Model file for the job. Use its own axes, mm. A direction names the side the tool comes from. Give positions to 0.01 mm unless a question says otherwise; leave off trailing zeros. Loops run counter-clockwise (first coordinate to the right, second up) from the corner with the lowest first, then second, coordinate; pieces in that order, holes last. Notation, with made-up numbers: (-28.75, -32.5) - (16.25, -32.5) arc R38 cw to (16.25, 5.5) - close; hole circle Ø9 at (86, 78). An arc over 180 degrees is marked (long way). Use a Markdown table: item, result.
Autodesk Inventor part; units mm, degrees
ref_plane "YZ Plane" through (0, 0, 0) normal (1, 0, 0) x (0, 1, 0)
ref_plane "XZ Plane" through (0, 0, 0) normal (0, 1, 0) x (-1, 0, 0)
ref_plane "XY Plane" through (0, 0, 0) normal (0, 0, 1) x (1, 0, 0)
sketch "Sketch1" plane through (0, 0, 0) normal (0, 1, 0) x (-1, 0, 0)
  line L0 (17, 5) -> (-17, 5)
  line L1 (-17, 5) -> (-17, -5)
  line L2 (-17, -5) -> (17, -5)
  line L3 (17, -5) -> (17, 5)
  line L4 (17, 5) -> (-17, -5) construction
  line L5 (-17, 5) -> (17, -5) construction
  point P0 (0, 0)
  dimension "d0" = 34
  dimension "d1" = 10
extrude "Extrusion1" add sketch "Sketch1" along normal blind 2.5
sketch "Sketch2" plane through (0, 2.5, 0) normal (0, 1, 0) x (1, 0, 0)
  line L0 (-17, 5) -> (-17, -5)
  circle A0 centre (-17, 0) radius 5
  line L1 (17, -5) -> (17, 5)
  circle A1 centre (17, 0) radius 5
  point P0 (0, 0)
extrude "Extrusion2" add sketch "Sketch2" against normal blind 2.5
sketch "Sketch3" plane through (0, 2.5, 0) normal (0, 1, 0) x (1, 0, 0)
  arc A0 (-17, 5) -> (-17, -5) centre (-17, 0) ccw
  circle A1 centre (-17, 0) radius 1.5
  arc A2 (17, -5) -> (17, 5) centre (17, 0) ccw
  circle A3 centre (17, 0) radius 1.5
  point P0 (0, 0)
  dimension "d6" = 3
  dimension "d7" = 3
hole "Hole1" at (-17, 2.5, 0) at (17, 2.5, 0) direction (0, -1, 0) diameter 2.85 end through all
sketch "Sketch4" plane through (0, 2.5, 0) normal (0, 1, 0) x (1, 0, 0)
  circle A0 centre (-17, 0) radius 4.25
  arc A1 (-17, 5) -> (-17, -5) centre (-17, 0) ccw
  arc A2 (17, -5) -> (17, 5) centre (17, 0) ccw
  circle A3 centre (17, 0) radius 4.25
  point P0 (0, 0)
  dimension "d15" = 8.5
  dimension "d16" = 8.5
extrude "Extrusion3" cut sketch "Sketch4" against normal blind 0.5
sketch "Sketch5" plane through (0, 2.5, 0) normal (0, 1, 0) x (1, 0, 0)
  circle A0 centre (0, 5) radius 1.5
  circle A1 centre (0, -5) radius 1.5
  circle A2 centre (0, 13.5) radius 10
  point P0 (0, 0)
  dimension "d19" = 3
  dimension "d20" = 5
  dimension "d21" = 3
  dimension "d22" = 5
  dimension "d23" = 20
extrude "Extrusion4" cut sketch "Sketch5" against normal through all contours A0 | A2
mirror "Mirror1" about plane through (0, 0, 0) normal (0, 0, 1) of "Extrusion4"
sketch "Sketch6" plane through (0, 2.5, 0) normal (0, 1, 0) x (1, 0, 0)
  circle A0 centre (6, 0) radius 3
  point P0 (0, 0)
  dimension "d26" = 6
  dimension "d27" = 6
extrude "Extrusion5" cut sketch "Sketch6" against normal blind 0.5
sketch "Sketch7" plane through (6, 2, 0) normal (0, 1, 0) x (1, 0, 0)
  circle A0 centre (0, 0) radius 3
  circle A1 centre (0, 0) radius 1.5
  point P0 (-6, 0)
  dimension "d30" = 3
extrude "Extrusion6" cut sketch "Sketch7" against normal through all contours A1
mirror "Mirror2" about plane through (0, 0, 0) normal (1, 0, 0) of "Extrusion5", "Extrusion6"
fillet "Fillet1" radius 4 4 edges at (5.2678, 1.25, 5) (-5.2678, 1.25, 5) (5.2678, 1.25, -5) (-5.2678, 1.25, -5)
properties part number "Tarot-mr4008-blade-adapter"
(1) Mould opens along X. For faces 1 (the flat face through (0, 0, 0)), 2 (the cylindrical face through (22, 1, 0)), 3 (the flat face through (-4.7, 2, 1.3)) say: pulls with the +X half, pulls with the -X half, needs draft (parallel to the pull), parting line crosses it, or undercut.
Computed:
| item | result |
|---|---|
| face 1 | needs draft |
| face 2 | pulls with the +X half |
| face 3 | undercut |
(2) Drill centre lines: probe 1 along X at (y, z) = (0.6, 0) (3 decimals); probe 2 along Z at (x, y) = (-17, 1.35) (3 decimals); probe 3 along Z at (x, y) = (-17, 2.45). Where is each one in solid material? Low to high. Write a range as [from, to].
Computed:
| item | result |
|---|---|
| probe 1 | [-22, -18.425], [-15.575, -7.5], [-4.5, 4.5], [7.5, 15.575], [18.425, 22] |
| probe 2 | [-5, -1.425], [1.425, 5] |
| probe 3 | [-5, -4.25], [4.25, 5] |
(3) Pin check, flat tip, straight feed: P1, Ø2.5, axis at x = -18.5, z = -0.5, coming from the +Y side. Stop position of the tip, or through.
Computed:
| item | result |
|---|---|
| P1 | y = 2 |
(4) Slice it at D-D, the plane z = -0.75. Count the separate pieces of the cut face and the enclosed holes in it, plus the area to 3 significant figures.
Computed:
| item | result |
|---|---|
| separate pieces | 5 |
| enclosed holes | 0 |
| area | 75.5 mm² |
(5) 3-axis set-ups, long thin cutter, end or side, ignore diameter. For faces 4 (the flat face through (-17, 2, 2)), 5 (the cylindrical face through (5.392, 1.268, -4.894)), 6 (the cylindrical face through (-5.392, 1.268, 4.894)): which of +Z, -Z, +X, -X, +Y, -Y reach the whole face in a straight line?
Computed:
| item | result |
|---|---|
| face 4 | +Y |
| face 5 | -Z, +Y, -Y |
| face 6 | +Z, +Y, -Y |
(6) Slice it at B-B, the plane x = 15. Write the cut outline in (y, z), plus the area to 4 significant figures.
Computed:
| item | result |
|---|---|
| outline | (0, -5) - (2.5, -5) - (2.5, -3.75) - (2, -3.75) - (2, 3.75) - (2.5, 3.75) - (2.5, 5) - (0, 5) - close |
| area | 21.25 mm² |
(7) Slice it at A-A, the plane y = 0.85. Write the cut outline in (x, z) (3 decimals), plus the area to 3 significant figures.
Computed:
| item | result |
|---|---|
| outline | (-17, -5) - (-6.305, -5) arc R4 ccw to (-4.503, -4.571) arc R10 cw to (4.503, -4.571) arc R4 ccw to (6.305, -5) - (17, -5) arc R5 ccw to (17, 5) - (6.305, 5) arc R4 ccw to (4.503, 4.571) arc R10 cw to (-4.503, 4.571) arc R4 ccw to (-6.305, 5) - (-17, 5) arc R5 ccw to start; hole circle Ø2.85 at (-17, 0); hole circle Ø3 at (-6, 0); hole circle Ø3 at (6, 0); hole circle Ø2.85 at (17, 0) |
| area | 370 mm² |
(8) Slice it at C-C, the plane z = 2.25. Write the cut outline in (x, y), plus the area to 3 significant figures.
Computed:
| item | result |
|---|---|
| outline | (-21.47, 0) - (21.47, 0) - (21.47, 2.5) - (20.61, 2.5) - (20.61, 2) - (13.39, 2) - (13.39, 2.5) - (7.98, 2.5) - (7.98, 2) - (4.02, 2) - (4.02, 2.5) - (-4.02, 2.5) - (-4.02, 2) - (-7.98, 2) - (-7.98, 2.5) - (-13.39, 2.5) - (-13.39, 2) - (-20.61, 2) - (-20.61, 2.5) - (-21.47, 2.5) - close |
| area | 96.1 mm² |
